Read the model definition and answer for the solid it produces. Units are mm, in the model's axes. A direction names the side the tool comes from. Give positions to 0.01 mm unless a question says otherwise; leave off trailing zeros. Order: outer loops, then holes, each group sorted by start corner. A loop starts at its lowest first (then second) coordinate and runs counter-clockwise, first axis right, second up. Notation, with made-up numbers: (10, 29) - (53, 29) arc R23 cw to (53, 59) - close; hole circle Ø8 at (28, 28). An arc over 180 degrees is marked (long way). Use a Markdown table: item, result. Add a question column.
1. A cutting plane is placed at A-A on z = -418. Determine the outline of the cut face in (x, y).
2. A cutting plane is placed at C-C on z = -588.5. Determine the outline of the cut face in (x, y), and give its area (3 significant figures).
3. Which of the six approach directions +Z, -Z, +X, -X, +Y, -Y give full straight-line access (tool end or side, diameter ignored) to faces 4 (the cylindrical face through (727.973, 0.732, -693.354)), 5 (the cylindrical face through (757.656, -0.732, -723.698))?
4. A cutting plane is placed at D-D on x = 288.5. Determine the outline of the cut face in (y, z).
5. Consider L1, parallel to X at y = 8.5, z = -481.5; L2, parallel to Z at x = -72.5, y = -10; L3, parallel to X at y = -37, z = -642. Determine where each line is inside the solid, lowest interval first.
6. For a pull along X with two mould halves and no side action, classify faces 1 (the flat face through (4, 52.308, -765)), 2 (the cylindrical face through (-727.973, 0.732, -693.354)), 3 (the flat face through (821.324, 1, -222)) as released by +X, released by -X, zero draft, split by the parting line, or undercut.
7. Flat-ended cylindrical pins translate along their axes: P1, Ø1.5, axis at y = -41, z = -628.5, coming from the -X side; P2, Ø10, axis at x = 413, y = -32.5, coming from the +Z side; P3, Ø5, axis at y = 10.5, z = -644, coming from the -X side. Find the tip coordinate at first contact, or state that the pin passes through.
8. A cutting plane is placed at B-B on y = -14. Determine the outline of the cut face in (x, z), and give its area (3 significant figures).
```python
from build123d import *

# Parameters (mm, degrees)
SKETCH2_W = 42.447903748
SKETCH2_H = 104.615154758


with BuildPart() as part:
    # Sweep1: sweep along a path in Sketch1
    with BuildLine(Plane(origin=(0, 0, 0), x_dir=(1, 0, 0), z_dir=(0, 1, 0))) as sweep1_path:
        Line((0, 762.84918933), (-609.6, 762.84918933))
        ThreePointArc((-609.6, 762.84918933), (-744.303841816, 707.053031146), (-800.1, 572.34918933))
        Line((-800.1, 572.34918933), (-800.1, -118.947967944))
    # Sketch2 → Sweep1 (sweep)
    with BuildSketch(Plane(origin=(-800.1, 0, 118.947967944), x_dir=(1, 0, 0), z_dir=(0, 0, 1))):
        Rectangle(SKETCH2_W, SKETCH2_H)
    sweep1 = sweep(path=sweep1_path.line)

    # Mirror1: Sweep1 across plane
    add(sweep1.mirror(Plane(origin=(0, 0, 37.25081067), x_dir=(0, 0, 1), z_dir=(1, 0, 0))))


solid = part.part
```
Output values:
| question | item | result |
|---|---|---|
| 1 | outline | (-821.32, -52.31) - (-778.88, -52.31) - (-778.88, 52.31) - (-821.32, 52.31) - close; (778.88, -52.31) - (821.32, -52.31) - (821.32, 52.31) - (778.88, 52.31) - close |
| 2 | outline | (-820.71, -52.31) - (-778.1, -52.31) - (-778.1, 52.31) - (-820.71, 52.31) - close; (778.1, -52.31) - (820.71, -52.31) - (820.71, 52.31) - (778.1, 52.31) - close |
| 2 | area | 8,910 mm² |
| 3 | face 4 | +Z, +Y, -Y |
| 3 | face 5 | -Z, +X, +Y, -Y |
| 4 | outline | (-52.31, -784.07) - (52.31, -784.07) - (52.31, -741.63) - (-52.31, -741.63) - close |
| 5 | L1 | -821.32 to -778.88, 778.88 to 821.32 |
| 5 | L2 | -784.07 to -741.63 |
| 5 | L3 | -809.54 to -763.88, 763.88 to 809.54 |
| 6 | face 1 | zero draft |
| 6 | face 2 | undercut |
| 6 | face 3 | released by +X |
| 7 | P1 | x = -813.95 |
| 7 | P2 | z = -741.63 |
| 7 | P3 | x = -809.71 |
| 8 | outline | (-821.32, -572.35) arc R211.72 ccw to (-609.6, -784.07) - (609.6, -784.07) arc R211.72 ccw to (821.32, -572.35) - (821.32, 118.95) - (778.88, 118.95) - (778.88, -572.35) arc R169.28 cw to (609.6, -741.63) - (-609.6, -741.63) arc R169.28 cw to (-778.88, -572.35) - (-778.88, 118.95) - (-821.32, 118.95) - close |
| 8 | area | 136,000 mm² |
